Source: three-view drawing plus pictorial views. Frame: mm from the lowest corner of the part. A direction names the side the tool comes from. Give positions to 0.01 mm unless a question says otherwise; leave off trailing zeros. Loops run counter-clockwise (first coordinate to the right, second up) from the corner with the lowest first, then second, coordinate; pieces in that order, holes last. Notation, with made-up numbers: (69, -35) - (89, -35) arc R27 cw to (89, -2) - close; hole circle Ø11 at (41.5, 18.25). An arc over 180 degrees is marked (long way). Write each question's results on one line, items separated by ' | '. Start each with the question number.
(1) Reachability of the marked faces 1 and 2 from +Z, -Z, +X, -X, +Y, -Y: full face, straight path, thin tool, end or side. Return the list, or none.
(2) Cut plane A-A on z = 37. Return the cut outline in (x, y) (1 decimal).
(3) Contact query for flat-ended pins moving along their axis: pin 1 (1.7 mm diameter, centred on y = 2, z = 51.5, fed in from +X) (1 decimal); pin 2 (2 mm diameter, centred on y = 4, z = 38.5, fed in from +X); pin 3 (1.5 mm diameter, centred on x = 22.5, y = 2.5, fed in from +Z). Output: stop coordinate, or through.
(4) Cut plane D-D on z = 46.5. Return the cut outline in (x, y), then the cut area to 3 significant figures.
(5) Material intervals for line 1 along X through (y, z) = (3.65, 49) (1 decimal); line 2 along X through (y, z) = (2.9, 54) (1 decimal); line 3 along Z through (x, y) = (53, 5.3) (1 decimal), sorted ascending. Write a range as [from, to].
(6) Cut plane B-B on x = 18.5. Return the cut outline in (y, z), then the cut area to 3 significant figures.
(7) Cut plane C-C on y = 3.5. Return the cut outline in (x, z).
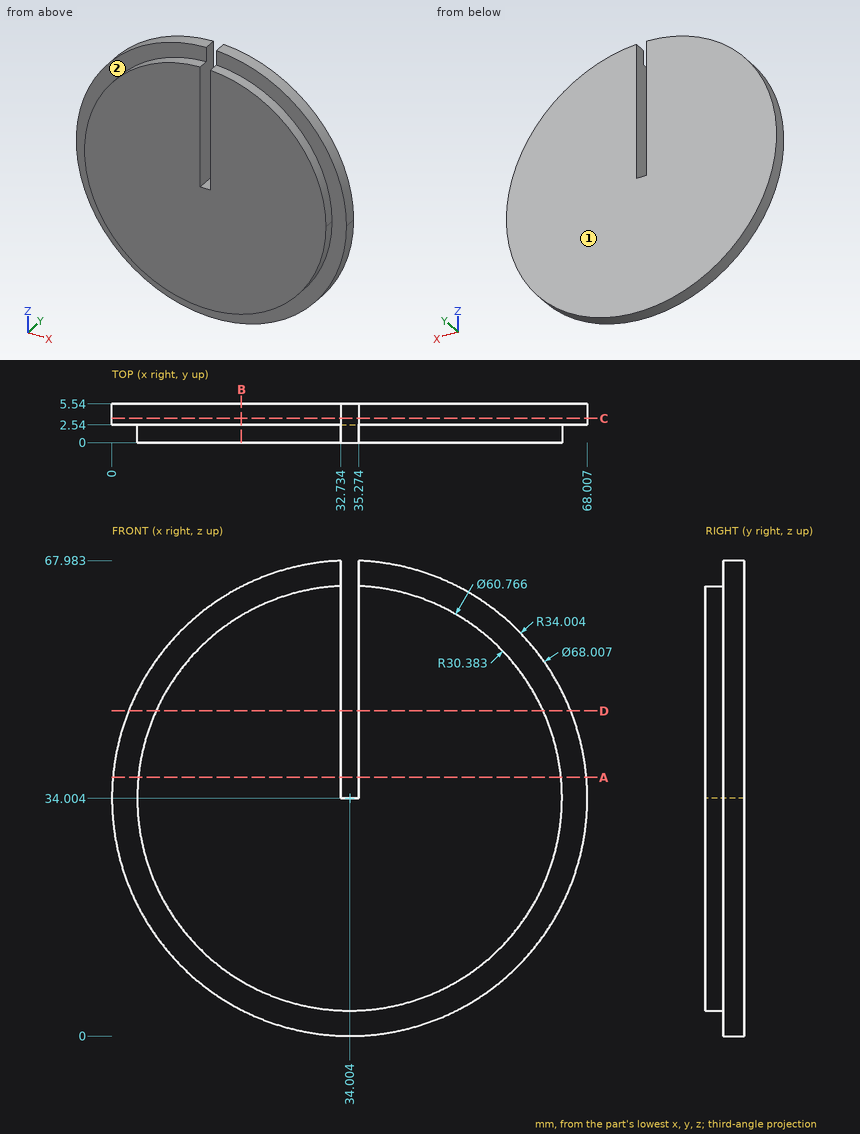
Ans:
1) face 1: +Z, -Z, +X, -X, +Y | face 2: -Y
2) outline: (0.1, 2.5) - (3.8, 2.5) - (3.8, 0) - (32.7, 0) - (32.7, 5.5) - (0.1, 5.5) - close; (35.3, 0) - (64.2, 0) - (64.2, 2.5) - (67.9, 2.5) - (67.9, 5.5) - (35.3, 5.5) - close
3) pin 1: x = 63.5 | pin 2: x = 67.83 | pin 3: z = 66.26
4) outline: (2.38, 2.54) - (6.31, 2.54) - (6.31, 0) - (32.73, 0) - (32.73, 5.54) - (2.38, 5.54) - close; (35.27, 0) - (61.7, 0) - (61.7, 2.54) - (65.63, 2.54) - (65.63, 5.54) - (35.27, 5.54) - close | area: 316 mm^2
5) line 1: [3.5, 32.7], [35.3, 64.5] | line 2: [6.5, 32.7], [35.3, 61.5] | line 3: [5.8, 62.2]
6) outline: (0, 7.87) - (2.54, 7.87) - (2.54, 3.74) - (5.54, 3.74) - (5.54, 64.27) - (2.54, 64.27) - (2.54, 60.13) - (0, 60.13) - close | area: 314 mm^2
7) outline: (32.73, 34) - (32.73, 67.98) arc R34 ccw (long way) to (35.27, 67.98) - (35.27, 34) - close
